```python
from build123d import *

# Parameters (mm, degrees)
EXTRUDE_1_DEPTH          = 55
CUT_EXTRUDE_3_DEPTH      = 323.664416923
PATTERN_CIRCULAR_1_COUNT = 8
CUT_EXTRUDE_4_DEPTH      = 158.777475037
PATTERN_CIRCULAR_2_COUNT = 8


with BuildPart() as part:
    # Sketch 1 → Extrude 1 (new body)
    with BuildSketch(Plane(origin=(0, 0, 0), x_dir=(1, 0, 0), z_dir=(0, 1, 0))):
        Polygon((42.426406871, -42.426406871), (60, 0), (42.426406871, 42.426406871), (0, 60), (-42.426406871, 42.426406871), (-60, 0), (-42.426406871, -42.426406871), (0, -60), align=None)
        Polygon((23.111992498, -9.573300746), (23.111992498, 9.573300746), (9.573300746, 23.111992498), (-9.573300746, 23.111992498), (-23.111992498, 9.573300746), (-23.111992498, -9.573300746), (-9.573300746, -23.111992498), (9.573300746, -23.111992498), align=None, mode=Mode.SUBTRACT)
    extrude(amount=EXTRUDE_1_DEPTH)

    # Sketch 4 → Cut-Extrude 3 (cut, through all, along a direction that is not the sketch's normal)
    with BuildSketch(Plane(origin=(-17.57970482, 20.884718614, 42.441161798), x_dir=(0.9373566365157255, 0.153814342715155, 0.31257588511436873), z_dir=(-0.34837126170211885, 0.4138656392921341, 0.8410426247422821))):
        Polygon((6.331993641, 36.93658877), (-26.507202364, -18.732285364), (18.754553107, -26.491452015), align=None)
    cut_extrude_3 = extrude(amount=CUT_EXTRUDE_3_DEPTH, dir=(0, 1, 0), mode=Mode.SUBTRACT)

    # Pattern Circular 1: Cut-Extrude 3 ×8 about axis
    pattern_circular_1_axis = Axis((0, 0, 0), (0, 1, 0))
    for i in range(1, PATTERN_CIRCULAR_1_COUNT):
        add(cut_extrude_3.rotate(pattern_circular_1_axis, i * 360 / PATTERN_CIRCULAR_1_COUNT), mode=Mode.SUBTRACT)

    # Sketch 8 → Cut-Extrude 4 (cut, through all, along a direction that is not the sketch's normal)
    with BuildSketch(Plane(origin=(-37.406700868, 47.713006316, 0), x_dir=(-0.7869756649359425, -0.616984037717858, 0), z_dir=(0.616984037717858, -0.7869756649359426, 0))):
        Polygon((-11.810668086, 11.644368558), (-11.810668086, -11.644368558), (28.709826154, 0), align=None)
    cut_extrude_4 = extrude(amount=-CUT_EXTRUDE_4_DEPTH, dir=(0, -1, 0), mode=Mode.SUBTRACT)

    # Pattern Circular 2: Cut-Extrude 4 ×8 about axis
    pattern_circular_2_axis = Axis((0, 0, 0), (0, 1, 0))
    for i in range(1, PATTERN_CIRCULAR_2_COUNT):
        add(cut_extrude_4.rotate(pattern_circular_2_axis, i * 360 / PATTERN_CIRCULAR_2_COUNT), mode=Mode.SUBTRACT)


solid = part.part
```
Work out the finished part from the listing and answer in its coordinate system (mm). A direction names the side the tool comes from. Coordinates: 2 decimals unless noted, no trailing zeros. Write each loop counter-clockwise with the first axis right and the second up, starting at its lowest first coordinate (ties: lowest second). Pieces come first, ordered by that corner, then holes.
Q1. Which of the six approach directions +Z, -Z, +X, -X, +Y, -Y give full straight-line access (tool end or side, diameter ignored) to faces 1 (the face through (-16.248, 27.115, -16.437)), 2 (the face through (-48.64, 31.05, 4.15)), 3 (the face through (16.8, 19.8, -43.3)), 4 (the face through (43.3, 19.8, 16.8))?
Q2. A cutting plane is placed at D-D, the plane x = 34. Give the vertices of the cut face in (y, z).
Q3. Each of these flat-tipped pins is pushed along its axis until it touches: pin 1 Ø3 at (x, y) = (28.5, 31) entering from -Z; pin 2 Ø1.5 at (y, z) = (36.5, 47.5) entering from -X; pin 3 Ø6 at (x, z) = (36.5, 0) entering from +Y. Where does it stop, or does it pass through?
Q4. A cutting plane is placed at A-A, the plane x = -21.5. Give the vertices of the cut face in (y, z).
Q5. A cutting plane is placed at B-B, the plane z = -5. Give the vertices of the cut face in (x, y).
Q6. Determine the mould class of faces 5 (the face through (-37.328, 31.046, -31.463)), 6 (the face through (-31.894, 30.276, -37.529)), 7 (the face through (37.529, 30.276, -31.894)) for opening direction X: released by +X, released by -X, zero draft, split by the parting line, or undercut.
Q7. Find the intervals of material crossed by line 1 (Z direction, x = -40.5, y = 31.5); line 2 (Z direction, x = 37, y = 38); line 3 (X direction, y = 31, z = -41), in increasing order.
Findings below:
1. face 1: +Y, -Y
1. face 2: +Z, -X, +Y
1. face 3: -Z, +Y
1. face 4: +X, +Y
2. outline: (0, -45.92) - (15.06, -38.51) - (36.84, -38.51) - (44.72, -24.31) - (32.38, -24.31) - (44.84, -9.49) - (50.38, -9.49) - (50.38, 9.49) - (44.84, 9.49) - (32.38, 24.31) - (44.72, 24.31) - (36.84, 38.51) - (15.06, 38.51) - (0, 45.92) - close
3. pin 1: stops at z = -36.65
3. pin 2: stops at x = -4.84
3. pin 3: stops at y = 50.78
4. outline: (0, -51.09) - (37.39, -32.7) - (47, -32.7) - (55, -18.26) - (55, -11.19) - (0, -11.19) - close; (0, 11.19) - (55, 11.19) - (55, 18.26) - (47, 32.7) - (37.39, 32.7) - (0, 51.09) - close
5. outline: (-57.93, 0) - (-23.11, 0) - (-23.11, 55) - (-28.11, 55) - (-46.31, 40.73) - (-46.31, 23.62) - close; (23.11, 0) - (57.93, 0) - (46.31, 23.62) - (46.31, 40.73) - (28.11, 55) - (23.11, 55) - close
6. face 5: released by -X
6. face 6: undercut
6. face 7: released by +X
7. line 1: z = -41.53 to -38.28, -9.66 to 9.66, 38.28 to 41.53
7. line 2: z = -33.42 to -30.76, -10.38 to 10.38, 30.76 to 33.42
7. line 3: x = -41.76 to -39.36, -9.04 to 9.04, 39.36 to 41.76
